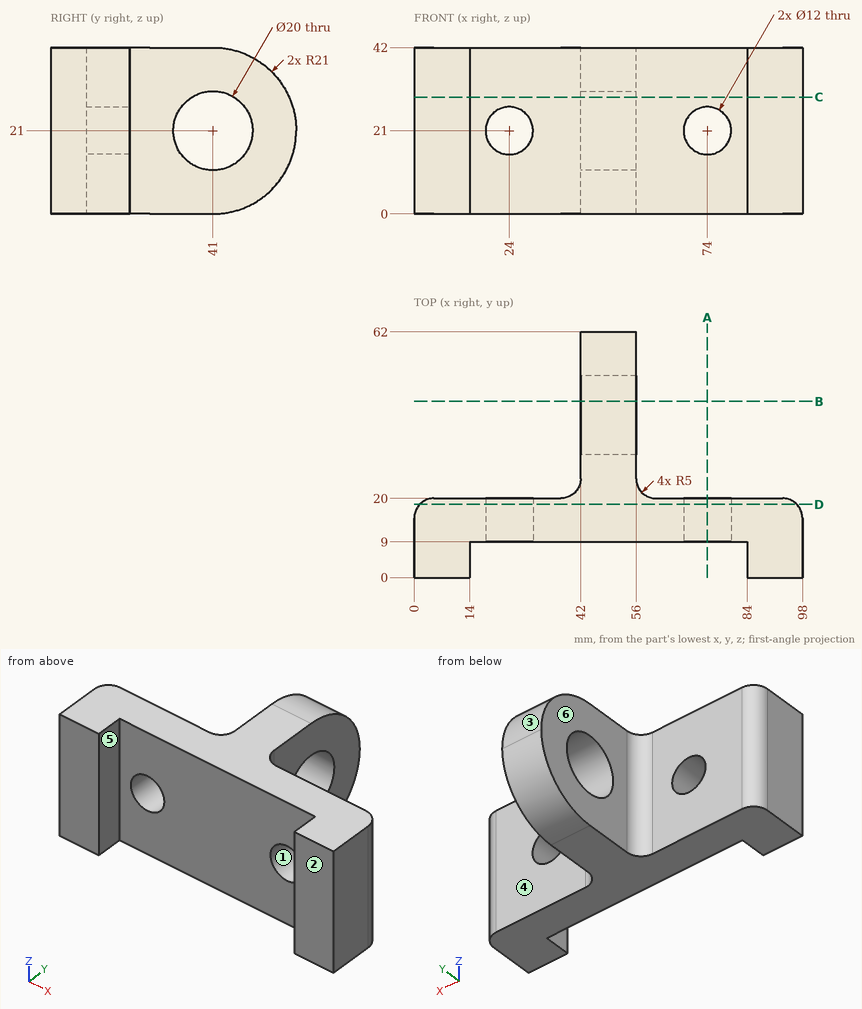
Job drawing, mm, ordinate dimensions from the low corner. One solid piece. A direction names the side the tool comes from. Coordinates: 2 decimals unless noted, no trailing zeros. Loops run counter-clockwise (first coordinate to the right, second up) from the corner with the lowest first, then second, coordinate; pieces in that order, holes last. Notation, with made-up numbers: (-38, 26) - (11, 26) arc R33 cw to (11, 61) - close; hole circle Ø10 at (-2, -11.5). An arc over 180 degrees is marked (long way). Answer as a JSON object with one key per item and string values. Group by question number.
(1) Cut at C-C (z = 29.5). Give the cut face in (x, y).
(2) Probe line 1 along X through (y, z) = (15, 21); line 2 along X through (y, z) = (7, 30.5); line 3 along Y through (x, z) = (46, 21). List the from-to ranges inside material, lowest first.
(3) Tool access for the marked faces 4, 5 and 6: list every direction of +Z, -Z, +X, -X, +Y, -Y with a clear straight run to the whole face (end or side of a thin tool).
(4) Cut at D-D (y = 18.5). Give the cut face in (x, z).
(5) Cut at B-B (y = 44.5). Give the cut face in (x, z).
(6) Two-plate mould, pull along Z, no slides. Class the marked faces 1, 2 and 3: released by +Z, released by -Z, zero draft, split by the parting line, or undercut.
(7) Flat gauge pins, fed straight in: pin 1 (11 mm diameter, centred on x = 74, z = 21, fed in from -Y); pin 2 (18.5 mm diameter, centred on y = 42.5, z = 30.5, fed in from -X); pin 3 (12 mm diameter, centred on x = 53.5, z = 9, fed in from +Y); pin 4 (4 mm diameter, centred on x = 52.5, y = 50, fed in from -Z). Where does each tip first touch, or does it go through?
(8) Cut at A-A (x = 74). Give the cut face in (y, z).
Geometry says:
{
 "1": {"outline": "(0, 0) - (14, 0) - (14, 9) - (84, 9) - (84, 0) - (98, 0) - (98, 15) arc R5 ccw to (93, 20) - (61, 20) arc R5 cw to (56, 25) - (56, 35.73) - (42, 35.73) - (42, 25) arc R5 cw to (37, 20) - (5, 20) arc R5 ccw to (0, 15) - close; (42, 46.27) - (56, 46.27) - (56, 60.2) - (42, 60.2) - close"},
 "2": {"line 1": "x = 0 to 18, 30 to 68, 80 to 98", "line 2": "x = 0 to 14, 84 to 98", "line 3": "y = 9 to 31, 51 to 62"},
 "3": {"face 4": "+Z, -Z, +X, +Y", "face 5": "+Z, -Z, -Y", "face 6": "+Z, -Z, -X, +Y"},
 "4": {"outline": "(1.43, 0) - (96.57, 0) - (96.57, 42) - (1.43, 42) - close; hole circle Ø12 at (24, 21); hole circle Ø12 at (74, 21)"},
 "5": {"outline": "(42, 0.29) - (56, 0.29) - (56, 11.63) - (42, 11.63) - close; (42, 30.37) - (56, 30.37) - (56, 41.71) - (42, 41.71) - close"},
 "6": {"face 1": "undercut", "face 2": "zero draft", "face 3": "released by +Z"},
 "7": {"pin 1": "passes through", "pin 2": "stops at x = 42", "pin 3": "stops at y = 61.12", "pin 4": "stops at z = 1.2"},
 "8": {"outline": "(9, 0) - (20, 0) - (20, 15) - (9, 15) - close; (9, 27) - (20, 27) - (20, 42) - (9, 42) - close"}
}
